from build123d import *

# Parameters (mm, degrees)
BOSS_EXTRUDE1_DEPTH     = 8
CUT_EXTRUDE1_REACH      = 47.847
SKETCH2_R               = 3.05
SKETCH5_R               = 2.7
BOSS_EXTRUDE2_DEPTH     = 5.5
SKETCH6_R               = 15.35
BOSS_EXTRUDE3_DEPTH     = 5.5
SKETCH7_R               = 5.5
CUT_EXTRUDE2_DEPTH      = 6.5
CUT_EXTRUDE3_DEPTH      = 52.305457799
CUT_EXTRUDE3_DEPTH_BACK = 52.305457799
SKETCH8_R               = 1.475


with BuildPart() as part:
    # Sketch1 → Boss-Extrude1 (new body)
    with BuildSketch(Plane.XY):
        with BuildLine():
            Line((28.511576596, -20.3), (22.2, -20.3))
            Line((22.2, -20.3), (22.2, 20.3))
            Line((22.2, 20.3), (28.511576596, 20.3))
            ThreePointArc((28.511576596, 20.3), (0, 35), (-28.511576596, 20.3))
            Line((-28.511576596, 20.3), (-22.2, 20.3))
            Line((-22.2, 20.3), (-22.2, -20.3))
            Line((-22.2, -20.3), (-28.511576596, -20.3))
            ThreePointArc((-28.511576596, -20.3), (0, -35), (28.511576596, -20.3))
        make_face()
    extrude(amount=BOSS_EXTRUDE1_DEPTH)

    # Sketch2 → Cut-Extrude1 (cut, up to next)
    with BuildSketch(Plane.XY.offset(8), mode=Mode.PRIVATE) as cut_extrude1_sk1:
        with Locations((17.67766953, -17.67766953)):
            Circle(SKETCH2_R)
    cut_extrude1_tool1 = extrude(cut_extrude1_sk1.sketch, amount=-CUT_EXTRUDE1_REACH, mode=Mode.PRIVATE) & part.part
    # Sketch2 → Cut-Extrude1 (cut, up to next)
    with BuildSketch(Plane.XY.offset(8), mode=Mode.PRIVATE) as cut_extrude1_sk2:
        with Locations((17.67766953, 17.67766953)):
            Circle(SKETCH2_R)
    cut_extrude1_tool2 = extrude(cut_extrude1_sk2.sketch, amount=-CUT_EXTRUDE1_REACH, mode=Mode.PRIVATE) & part.part
    # Sketch2 → Cut-Extrude1 (cut, up to next)
    with BuildSketch(Plane.XY.offset(8), mode=Mode.PRIVATE) as cut_extrude1_sk3:
        with Locations((-17.67766953, 17.67766953)):
            Circle(SKETCH2_R)
    cut_extrude1_tool3 = extrude(cut_extrude1_sk3.sketch, amount=-CUT_EXTRUDE1_REACH, mode=Mode.PRIVATE) & part.part
    # Sketch2 → Cut-Extrude1 (cut, up to next)
    with BuildSketch(Plane.XY.offset(8), mode=Mode.PRIVATE) as cut_extrude1_sk4:
        with Locations((-17.67766953, -17.67766953)):
            Circle(SKETCH2_R)
    cut_extrude1_tool4 = extrude(cut_extrude1_sk4.sketch, amount=-CUT_EXTRUDE1_REACH, mode=Mode.PRIVATE) & part.part
    add(cut_extrude1_tool1.solids().sort_by_distance((17.67767, -17.67767, 8))[0], mode=Mode.SUBTRACT)
    add(cut_extrude1_tool2.solids().sort_by_distance((17.67767, 17.67767, 8))[0], mode=Mode.SUBTRACT)
    add(cut_extrude1_tool3.solids().sort_by_distance((-17.67767, 17.67767, 8))[0], mode=Mode.SUBTRACT)
    add(cut_extrude1_tool4.solids().sort_by_distance((-17.67767, -17.67767, 8))[0], mode=Mode.SUBTRACT)

    # Sketch5 → Boss-Extrude2 (add)
    with BuildSketch(Plane.XY.offset(8)):
        with BuildLine():
            ThreePointArc((-24.477540726, -20.3), (-31.8, 0), (-24.477540726, 20.3))
            Line((-24.477540726, 20.3), (-28.511576596, 20.3))
            ThreePointArc((-28.511576596, 20.3), (-35, 0), (-28.511576596, -20.3))
            Line((-28.511576596, -20.3), (-24.477540726, -20.3))
        make_face()
        with BuildLine():
            ThreePointArc((-24.477540726, 20.3), (0, 31.8), (24.477540726, 20.3))
            Line((24.477540726, 20.3), (28.511576596, 20.3))
            ThreePointArc((28.511576596, 20.3), (0, 35), (-28.511576596, 20.3))
            Line((-28.511576596, 20.3), (-24.477540726, 20.3))
        make_face()
        with BuildLine():
            ThreePointArc((24.477540726, 20.3), (29.913423367, 10.79013913), (31.8, 0))
            ThreePointArc((31.8, 0), (29.913423367, -10.79013913), (24.477540726, -20.3))
            Line((24.477540726, -20.3), (28.511576596, -20.3))
            ThreePointArc((28.511576596, -20.3), (33.33845513, -10.655862685), (35, 0))
            ThreePointArc((35, 0), (33.33845513, 10.655862685), (28.511576596, 20.3))
            Line((28.511576596, 20.3), (24.477540726, 20.3))
        make_face()
        with BuildLine():
            Line((28.511576596, -20.3), (24.477540726, -20.3))
            ThreePointArc((24.477540726, -20.3), (0, -31.8), (-24.477540726, -20.3))
            Line((-24.477540726, -20.3), (-28.511576596, -20.3))
            ThreePointArc((-28.511576596, -20.3), (0, -35), (28.511576596, -20.3))
        make_face()
        with Locations((0, 25)):
            Circle(SKETCH5_R)
    extrude(amount=BOSS_EXTRUDE2_DEPTH)

    # Sketch6 → Boss-Extrude3 (add)
    with BuildSketch(Plane.XY.offset(8)):
        with Locations(Location((0, 0, 0), (0, 0, 180))):
            Circle(SKETCH6_R)
    extrude(amount=BOSS_EXTRUDE3_DEPTH)

    # Sketch7 → Cut-Extrude2 (cut)
    with BuildSketch(Plane(origin=(0, 0, 0), x_dir=(-1, 0, 0), z_dir=(0, 0, -1))):
        with Locations((-17.67766953, 17.67766953)):
            Circle(SKETCH7_R)
        with Locations((17.67766953, 17.67766953)):
            Circle(SKETCH7_R)
        with Locations((17.67766953, -17.67766953)):
            Circle(SKETCH7_R)
        with Locations((-17.67766953, -17.67766953)):
            Circle(SKETCH7_R)
    extrude(amount=-CUT_EXTRUDE2_DEPTH, mode=Mode.SUBTRACT)

    # Sketch8 → Cut-Extrude3 (cut, two sides: drawn at the far end of the back side and taken through both)
    with BuildSketch(Plane(origin=(0, 0, 0), x_dir=(0, 0, -1), z_dir=(1, 0, 0)).offset(-CUT_EXTRUDE3_DEPTH_BACK)):
        with Locations(Location((-4, 7.5, 0), (0, 0, 90))):
            Circle(SKETCH8_R)
        with Locations(Location((-4, -7.5, 0), (0, 0, 90))):
            Circle(SKETCH8_R)
    extrude(amount=CUT_EXTRUDE3_DEPTH + CUT_EXTRUDE3_DEPTH_BACK, mode=Mode.SUBTRACT)


solid = part.part
The model under review builds one solid part; all positions refer to its coordinate system, in mm. A direction names the side the tool comes from. Give positions to 0.01 mm unless a question says otherwise; leave off trailing zeros. Loops run counter-clockwise (first coordinate to the right, second up) from the corner with the lowest first, then second, coordinate; pieces in that order, holes last. Notation, with made-up numbers: (-20, 58.5) -> (21, 58.5) arc R6 cw to (21, 63.5) -> close; hole circle Ø4 at (74.5, -4). An arc over 180 degrees is marked (long way). Answer as a JSON object with one key per item and string values. Group by question number.
Q1. Take a section at A-A (z = 9.5). Write out the cut boundary in (x, y), plus the area to 3 significant figures.
Q2. Insertion check: pin 1 (3 mm diameter, centred on y = -6, z = 8, fed in from +X); pin 2 (6 mm diameter, centred on x = -8.5, y = 21.5, fed in from +Z); pin 3 (2 mm diameter, centred on y = 11.5, z = 10, fed in from +X). Each pin has a flat end and moves straight along its axis. Give the tip position at first contact, or say it passes through.
Q3. Take a section at D-D (x = 0). Write out the cut boundary in (y, z) (3 decimals).
Q4. Wall thickness on line 1 along Y through (x, z) = (10.5, 4) (3 decimals); line 2 along Y through (x, z) = (18, 5.25); line 3 along Y through (x, z) = (-2, 4) (3 decimals): over which ranges is each line inside the solid? List them lowest first.
Q5. Take a section at B-B (x = -17.5). State how many separate pieces and enclosed holes the cut face has, plus the area to 3 significant figures.
Q6. Tool access review of faces 4 (the flat face through (-20, -15, 6.5)), 5 (the cylindrical face through (-7.08, 13.62, 10.71)), 6 (the flat face through (25, 20.3, 4)): name each direction out of +Z, -Z, +X, -X, +Y, -Y from which nothing blocks a thin tool from reaching the whole face with its end or side.
Q7. Take a section at C-C (y = 2.5). Write out the cut boundary in (x, z), plus the area to 3 significant figures.
Q8. Draft analysis for pull direction Y (two halves, no side actions). For faces 1 (the flat face through (32, 0, 8)), 2 (the flat face through (0, 0, 13.5)), 3 (the flat face through (-22.2, 0, 4)), state which applies: pulls with the +Y half, pulls with the -Y half, needs draft (parallel to the pull), parting line crosses it, or undercut.
Answer below:
{
 "1": {"outline": "circle Ø70 at (0, 0); circle Ø30.7 at (0, 0); circle Ø5.4 at (0, 25); hole circle Ø63.6 at (0, 0)", "area": "1,430 mm2"},
 "2": {"pin 1": "stops at x = 34.71", "pin 2": "stops at z = 8", "pin 3": "stops at x = 33.39"},
 "3": {"outline": "(-35, 0) -> (35, 0) -> (35, 13.5) -> (31.8, 13.5) -> (31.8, 8) -> (27.7, 8) -> (27.7, 13.5) -> (22.3, 13.5) -> (22.3, 8) -> (15.35, 8) -> (15.35, 13.5) -> (-15.35, 13.5) -> (-15.35, 8) -> (-31.8, 8) -> (-31.8, 13.5) -> (-35, 13.5) -> close; hole circle Ø2.95 at (-7.5, 4); hole circle Ø2.95 at (7.5, 4)"},
 "4": {"line 1": "y = -33.388 to -8.975, -6.025 to 6.025, 8.975 to 33.388", "line 2": "y = -30.02 to -23.17, -12.19 to -8.28, -6.72 to 6.72, 8.28 to 12.19, 23.17 to 30.02", "line 3": "y = -34.943 to -8.975, -6.025 to 6.025, 8.975 to 34.943"},
 "5": {"separate pieces": "3", "enclosed holes": "2", "area": "351 mm2"},
 "6": {"face 4": "-Z", "face 5": "+Z", "face 6": "-Z, +X"},
 "7": {"outline": "(-34.91, 8) -> (-31.7, 8) -> (-31.7, 13.5) -> (-34.91, 13.5) -> close; (-22.2, 0) -> (22.2, 0) -> (22.2, 8) -> (15.15, 8) -> (15.15, 13.5) -> (-15.15, 13.5) -> (-15.15, 8) -> (-22.2, 8) -> close; (31.7, 8) -> (34.91, 8) -> (34.91, 13.5) -> (31.7, 13.5) -> close", "area": "557 mm2"},
 "8": {"face 1": "undercut", "face 2": "needs draft", "face 3": "undercut"}
}
